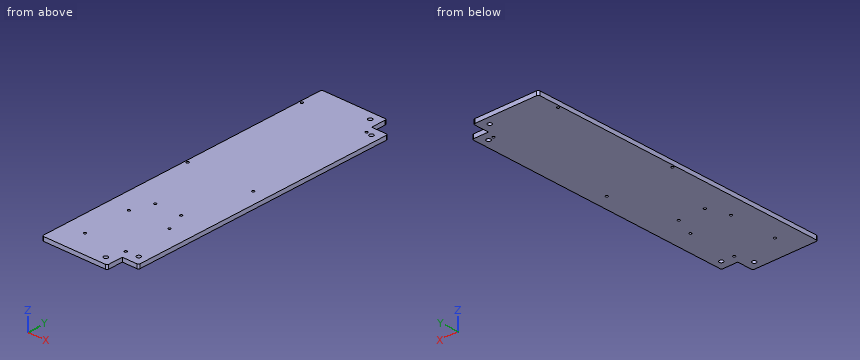
from build123d import *

# Parameters (mm, degrees)
SKETCH_2_W          = 100
SKETCH_2_H          = 370
EXTRUDE_1_DEPTH     = 2.5
SKETCH_5_R          = 1.5
CUT_EXTRUDE_3_DEPTH = 192.702895127
SKETCH_6_R          = 1.5
CUT_EXTRUDE_4_DEPTH = 192.702895127
SKETCH_7_W          = 20
SKETCH_7_H          = 20
CUT_EXTRUDE_5_DEPTH = 192.702895127
SKETCH_8_R          = 2.55
CUT_EXTRUDE_6_DEPTH = 192.702895127
FILLET_1_R          = 2
SKETCH_10_R         = 1.5
CUT_EXTRUDE_7_DEPTH = 13


with BuildPart() as part:
    # 草图2 → 凸台-拉伸1 (new, symmetric)
    with BuildSketch(Plane.XY):
        Rectangle(SKETCH_2_W, SKETCH_2_H)
    extrude(amount=EXTRUDE_1_DEPTH, both=True)

    # 草图5 → 切除-拉伸3 (cut, through all)
    with BuildSketch(Plane.XY.offset(2.5)):
        with Locations((33, 155)):
            Circle(SKETCH_5_R)
        with Locations(Location((-47, 155.654762379, 0), (0, 0, 180))):
            Circle(SKETCH_5_R)
        with Locations(Location((33, 5, 0), (0, 0, 180))):
            Circle(SKETCH_5_R)
        with Locations((-47, 4.345237621)):
            Circle(SKETCH_5_R)
    extrude(amount=-CUT_EXTRUDE_3_DEPTH, mode=Mode.SUBTRACT)

    # 草图6 → 切除-拉伸4 (cut, through all)
    with BuildSketch(Plane.XY.offset(2.5)):
        with Locations((25, -155)):
            Circle(SKETCH_6_R)
        with Locations(Location((-25, -155, 0), (0, 0, 180))):
            Circle(SKETCH_6_R)
        with Locations(Location((25, -97, 0), (0, 0, 180))):
            Circle(SKETCH_6_R)
        with Locations((-25, -97)):
            Circle(SKETCH_6_R)
    extrude(amount=-CUT_EXTRUDE_4_DEPTH, mode=Mode.SUBTRACT)

    # 草图7 → 切除-拉伸5 (cut, through all)
    with BuildSketch(Plane.XY.offset(2.5)):
        with Locations((40, 175)):
            Rectangle(SKETCH_7_W, SKETCH_7_H)
        with Locations((40, -175)):
            Rectangle(SKETCH_7_W, SKETCH_7_H)
    extrude(amount=-CUT_EXTRUDE_5_DEPTH, mode=Mode.SUBTRACT)

    # 草图8 → 切除-拉伸6 (cut, through all)
    with BuildSketch(Plane(origin=(0, 0, -2.5), x_dir=(-1, 0, 0), z_dir=(0, 0, -1))):
        with Locations((-19, 175)):
            Circle(SKETCH_8_R)
        with Locations((-40, 154)):
            Circle(SKETCH_8_R)
        with Locations((-40, -154)):
            Circle(SKETCH_8_R)
        with Locations((-19, -175)):
            Circle(SKETCH_8_R)
    extrude(amount=-CUT_EXTRUDE_6_DEPTH, mode=Mode.SUBTRACT)

    # 圆角1
    fillet_1_edges = [part.edges().sort_by_distance(p)[0] for p in [
        (50, 165, 0),
        (30, 185, 0),
        (30, -185, 0),
        (50, -165, 0),
        (-50, 185, 0),
        (-50, -185, 0),
    ]]
    fillet(fillet_1_edges, radius=FILLET_1_R)

    # 草图10 → 切除-拉伸7 (cut)
    with BuildSketch(Plane(origin=(0, 0, -2.5), x_dir=(-1, 0, 0), z_dir=(0, 0, -1))):
        with Locations((-16, -72)):
            Circle(SKETCH_10_R)
        with Locations((16, -72)):
            Circle(SKETCH_10_R)
    extrude(amount=-CUT_EXTRUDE_7_DEPTH, mode=Mode.SUBTRACT)


solid = part.part
Verification items for the finished model (mm, model axes). Give positions to 0.01 mm unless a question says otherwise; leave off trailing zeros. Answer as a JSON object with one key per item and string values. Group by question number.
1) Scan lines: line 1 along X through (y, z) = (-97, -0.8); line 2 along Y through (x, z) = (19, -1.3); line 3 along Y through (x, z) = (40, 0.95). Record each from-to range of solid material in increasing order. Write a range as [from, to].
2) Depth check by flat-ended pin: pin 1 Ø2.5 at (x, y) = (-25, -97) entering from -Z; pin 2 Ø1.5 at (y, z) = (-177.5, 0) entering from +X. Enter the tip coordinate at first touch or a pass-through.
3) Cross-section at A-A (z = 1.15). Give the number of separate pieces and of enclosed holes in the cut face, then the cut area to 3 significant figures.
Result sheet:
{
 "1": {"line 1": "x = [-50, -26.5], [-23.5, 23.5], [26.5, 50]", "line 2": "y = [-185, -177.55], [-172.45, 172.45], [177.55, 185]", "line 3": "y = [-165, -156.55], [-151.45, 151.45], [156.55, 165]"},
 "2": {"pin 1": "passes through", "pin 2": "stops at x = 30"},
 "3": {"separate pieces": "1", "enclosed holes": "14", "area": "36,000 mm2"}
}
